from build123d import *

# Parameters (mm, degrees)
SALIENTE_EXTRUIR1_DEPTH      = 6.35
TALADRO_DE_MARGEN_PARA_M41_D = 4.5
REDONDEO1_R                  = 5


# Read off the part's stored shape, not the designer's step: Saliente-Extruir1
with BuildPart() as part:
    # Saliente-Extruir1 outline → Saliente-Extruir1 (new body)
    with BuildSketch(Plane(origin=(0, 0, 0), x_dir=(0, 0, -1), z_dir=(1, 0, 0))):
        with BuildLine():
            Line((-2.5, 180), (-17.5, 180))
            Line((-17.5, 180), (-17.5, 100))
            add(Edge.make_bspline(
                [(-17.5, 100), (-17.5, 98.712751966), (-17.500047788, 96.116321069), (-17.51148981, 91.098940131), (-17.565479393, 85.046877218), (-17.737925717, 78.203948852), (-18.147729277, 69.656133307), (-19.038911227, 60.095322328), (-20.718334539, 50.310614009), (-22.956153632, 41.771686415), (-25.785586207, 33.773608765), (-29.338865081, 25.548124026), (-33.697565336, 16.449967912), (-38.713561507, 6.016494532), (-43.953609584, -6.016361906), (-48.809754323, -19.661313126), (-52.733015331, -34.671033487), (-55.439087369, -50.654463146), (-56.694005293, -64.452671708), (-57.222054598, -75.565918854), (-57.428472519, -83.87427142), (-57.487938926, -90.701655992), (-57.499988878, -96.070691027), (-57.5, -98.684323127), (-57.5, -100)],
                knots=[0, 0, 0, 0, 0.015625, 0.03125, 0.0625, 0.09375, 0.125, 0.1875, 0.25, 0.3125, 0.375, 0.4375, 0.5, 0.5625, 0.625, 0.6875, 0.75, 0.8125, 0.875, 0.90625, 0.9375, 0.96875, 0.984375, 1, 1, 1, 1], degree=3))
            Line((-57.5, -100), (-57.5, -180))
            Line((-57.5, -180), (-42.5, -180))
            Line((-42.5, -180), (-42.5, -150))
            Line((-42.5, -150), (2.5, -150))
            Line((2.5, -150), (2.5, -180))
            Line((2.5, -180), (17.5, -180))
            Line((17.5, -180), (17.5, -100))
            add(Edge.make_bspline(
                [(17.5, -100), (17.5, -98.712751966), (17.500047788, -96.116321069), (17.51148981, -91.098940131), (17.565479393, -85.046877218), (17.737925717, -78.203948852), (18.147729277, -69.656133307), (19.038911227, -60.095322328), (20.718334539, -50.310614009), (22.956153632, -41.771686415), (25.785586207, -33.773608765), (29.338865081, -25.548124026), (33.697565336, -16.449967912), (38.713561507, -6.016494532), (43.953609584, 6.016361906), (48.809754323, 19.661313126), (52.733015331, 34.671033487), (55.439087369, 50.654463146), (56.694005293, 64.452671708), (57.222054598, 75.565918854), (57.428472519, 83.87427142), (57.487938926, 90.701655992), (57.499988878, 96.070691027), (57.5, 98.684323127), (57.5, 100)],
                knots=[0, 0, 0, 0, 0.015625, 0.03125, 0.0625, 0.09375, 0.125, 0.1875, 0.25, 0.3125, 0.375, 0.4375, 0.5, 0.5625, 0.625, 0.6875, 0.75, 0.8125, 0.875, 0.90625, 0.9375, 0.96875, 0.984375, 1, 1, 1, 1], degree=3))
            Line((57.5, 100), (57.5, 180))
            Line((57.5, 180), (42.5, 180))
            Line((42.5, 180), (42.5, 150))
            Line((42.5, 150), (-2.5, 150))
            Line((-2.5, 150), (-2.5, 180))
        make_face()
    extrude(amount=SALIENTE_EXTRUIR1_DEPTH)

    # Taladro de margen para M41 (through all)
    with Locations(Plane.ZY):
        with Locations((10, 163), (10, 175), (-50, 163), (-50, 175), (50, -175), (50, -163), (-10, -175), (-10, -163), (-2.5, 85), (-2.5, 73), (-37.5, 73), (-37.5, 85)):
            Hole(TALADRO_DE_MARGEN_PARA_M41_D / 2)

    # Redondeo1
    redondeo1_edges = [part.edges().sort_by_distance(p)[0] for p in [
        (3.175, 180, 2.5),
        (3.175, 180, -42.5),
        (3.175, 180, -57.5),
        (3.175, -180, -17.5),
        (3.175, -180, -2.5),
        (3.175, -180, 42.5),
        (3.175, -180, 57.5),
        (3.175, 180, 17.5),
    ]]
    fillet(redondeo1_edges, radius=REDONDEO1_R)


solid = part.part
Source: CAD feature listing. Evaluate the final solid. Frame: model axes, mm. A direction names the side the tool comes from. Coordinates: 2 decimals unless noted, no trailing zeros. Write each loop counter-clockwise with the first axis right and the second up, starting at its lowest first coordinate (ties: lowest second). Pieces come first, ordered by that corner, then holes. Notation, with made-up numbers: M 32.5,-18.75 L 50.5,-18.75 A27 cw 50.5,-1.75 Z; hole C -21.5,65 d4. An arc over 180 degrees is marked long. Use a Markdown table: item, result.
1) Ray query, L1, parallel to Z at x = 3.5, y = 175; L2, parallel to Y at x = 2, z = -10; L3, parallel to Z at x = 1.75, y = 151.5. Return the intervals inside material, ascending.
Conclusion:
| item | result |
|---|---|
| L1 | z = -57.5 to -52.25, -47.75 to -42.5, 2.5 to 7.75, 12.25 to 17.5 |
| L2 | y = -180 to -177.25, -172.75 to -165.25, -160.75 to 150 |
| L3 | z = -57.5 to -42.5, 2.5 to 17.5 |
2) First-contact query: pin 1 Ø6 at (y, z) = (85, -37.5) entering from +X; pin 2 Ø3 at (x, z) = (2, -15) entering from +Y; pin 3 Ø3 at (x, y) = (4.5, 21) entering from -Z; pin 4 Ø4 at (y, z) = (163, 10) entering from -X. Flat tips, straight axial feed; report the tip coordinate or a pass-through.
Conclusion:
| item | result |
|---|---|
| pin 1 | stops at x = 6.35 |
| pin 2 | stops at y = 150 |
| pin 3 | stops at z = -49.43 |
| pin 4 | passes through |
3) Reachability of faces 1 (the flat face through (3, -138, -17.5)), 2 (the flat face through (3, 162, 2.5)), 3 (the flat face through (3, 138, 17.5)), 4 (the flat face through (3, -162, -2.5)) from +Z, -Z, +X, -X, +Y, -Y: full face, straight path, thin tool, end or side. Return the list, or none.
Conclusion:
| item | result |
|---|---|
| face 1 | -Z, +X, -X, -Y |
| face 2 | +X, -X, +Y |
| face 3 | +Z, +X, -X, +Y |
| face 4 | +X, -X, -Y |
4) Section B-B, the plane y = 135. Output: boundary loops of the cut face in (x, z), then the cut area to 3 significant figures.
Conclusion:
| item | result |
|---|---|
| outline | M 0,-57.5 L 6.35,-57.5 L 6.35,17.5 L 0,17.5 Z |
| area | 476 mm^2 |
5) Section A-A, the plane x = 2.75. Give the number of separate pieces and of enclosed holes in the cut face, then the cut area to 3 significant figures.
Conclusion:
| item | result |
|---|---|
| separate pieces | 1 |
| enclosed holes | 12 |
| area | 24,600 mm^2 |
6) Mould query, pull axis Z, two halves, no side actions, for faces 5 (the flat face through (3, -163, 42.5)), 6 (the flat face through (3, -137, 57.5)), 7 (the flat face through (0, 3, 1)). Classes: pulls with the +Z half, pulls with the -Z half, needs draft (parallel to the pull), parting line crosses it, or undercut.
Conclusion:
| item | result |
|---|---|
| face 5 | undercut |
| face 6 | pulls with the +Z half |
| face 7 | needs draft |
